Can you work these out from the model? Positions are in its coordinate system, mm. A direction names the side the tool comes from. Give positions to 0.01 mm unless a question says otherwise; leave off trailing zeros. Order: outer loops, then holes, each group sorted by start corner. A loop starts at its lowest first (then second) coordinate and runs counter-clockwise, first axis right, second up. Notation, with made-up numbers: (-40, 54.25) - (12, 54.25) arc R10 ccw to (12, 69.25) - close; hole circle Ø11 at (-35, -30). An arc over 180 degrees is marked (long way). Use one line per item in the form item = value. Start each with the question number.
1) Suppose I cut it at D-D, the plane z = -6.5. Write out the boundary of the cut face in (x, y).
2) We'd pull the mould along X, two halves only. Please class faces 3 (the cylindrical face through (58.72, -12.65, 8.06)), 4 (the flat face through (117, 4, 0)), 5 (the cylindrical face through (1.972, -12.165, -13.267)): released by +X, released by -X, zero draft, split by the parting line, or undercut.
3) For pin 1 (8 mm diameter, centred on x = 89, y = -4.5, fed in from +Z); pin 2 (3 mm diameter, centred on x = 68.5, z = 10, fed in from -Y); pin 3 (1 mm diameter, centred on y = 14, z = -14, fed in from -X); pin 4 (4 mm diameter, centred on x = 57.5, z = -4.5, fed in from -Y), each with a flat end and sliding along its axis, tell me the tip position at first contact or that it passes through.
4) Suppose I cut it at A-A, the plane y = 0. Write out the boundary of the cut face in (x, z), and give its area (3 significant figures).
5) Please list where these lines run through material, in increasing order: probe 1 along Y at (x, z) = (25, 0); probe 2 along X at (y, z) = (5, 15.5); probe 3 along Z at (x, y) = (92.5, -0.5).
6) Suppose I cut it at C-C, the plane x = 12. Write out the boundary of the cut face in (y, z).
7) Which directions (+Z, -Z, +X, -X, +Y, -Y) give clear straight access to the entire face, cutting with the end or side of a thin tool? Please do faces 1 (the cylindrical face through (57.68, 2.23, -0.29)), 2 (the flat face through (115, -15, -4)).
```python
from build123d import *

# Parameters (mm, degrees)
ESQUISSE4_R             = 2.25
ENL_V_MAT_EXTRU_2_DEPTH = 120.737212261


with BuildPart() as part:
    # Esquisse2 → Révolution1 (revolve)
    with BuildSketch(Plane.XY, mode=Mode.PRIVATE) as r_volution1_sk:
        Polygon((4, 18), (0, 18), (0, 0), (117, 0), (117, 18), (115, 18), (115, 15), (4, 15), align=None)
    revolve(r_volution1_sk.sketch.rotate(Axis((-23.43828007, 0, 0), (1, 0, 0)), 90), axis=Axis((-23.43828007, 0, 0), (1, 0, 0)))

    # Esquisse4 → Enlèv. mat.-Extru.2 (cut, through all)
    with BuildSketch(Plane.ZY):
        Circle(ESQUISSE4_R)
    extrude(amount=-ENL_V_MAT_EXTRU_2_DEPTH, mode=Mode.SUBTRACT)


solid = part.part
```
Result sheet:
q1.outline = (0, -16.79) - (4, -16.79) - (4, -13.52) - (115, -13.52) - (115, -16.79) - (117, -16.79) - (117, 16.79) - (115, 16.79) - (115, 13.52) - (4, 13.52) - (4, 16.79) - (0, 16.79) - close
q2.face_3 = undercut
q2.face_4 = released by +X
q2.face_5 = zero draft
q3.pin_1 = 14.99
q3.pin_2 = -12.36
q3.pin_3 = through
q3.pin_4 = -14.79
q4.outline = (0, -18) - (4, -18) - (4, -15) - (115, -15) - (115, -18) - (117, -18) - (117, -2.25) - (0, -2.25) - close; (0, 2.25) - (117, 2.25) - (117, 18) - (115, 18) - (115, 15) - (4, 15) - (4, 18) - (0, 18) - close
q4.area = 3,020 mm²
q5.probe_1 = -15 to -2.25, 2.25 to 15
q5.probe_2 = 0 to 4, 115 to 117
q5.probe_3 = -14.99 to -2.19, 2.19 to 14.99
q6.outline = circle Ø30 at (0, 0); hole circle Ø4.5 at (0, 0)
q7.face_1 = +X, -X
q7.face_2 = none
